Design review of the part shown in the three views and the two pictorial views. Dimensions are in mm from the part's minimum x, y and z. A direction names the side the tool comes from. Coordinates: 2 decimals unless noted, no trailing zeros. Write each loop counter-clockwise with the first axis right and the second up, starting at its lowest first coordinate (ties: lowest second). Pieces come first, ordered by that corner, then holes. Notation, with made-up numbers: (58.5, 37) -> (65.5, 37) arc R9 ccw to (65.5, 50) -> close; hole circle Ø8 at (-6.75, 6). An arc over 180 degrees is marked (long way). Write each question's results on one line, items separated by ' | '.
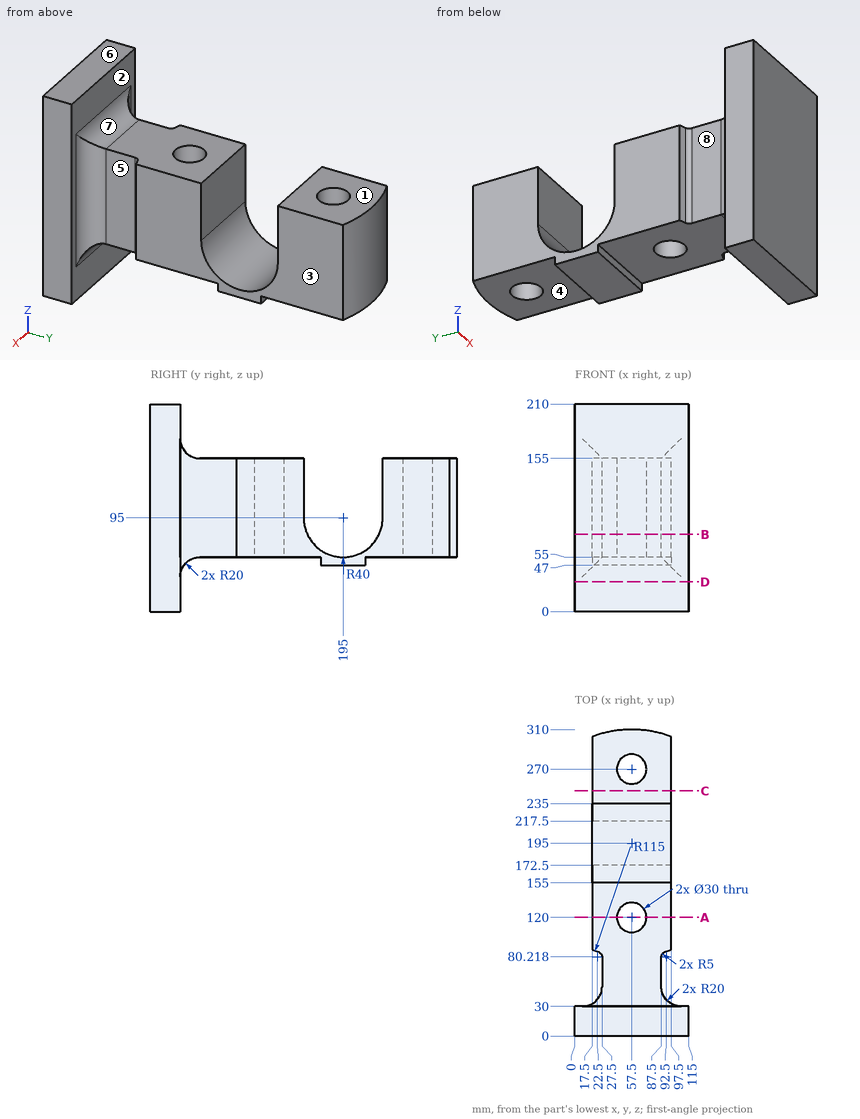
Q1. Add section A-A (y = 120). Write out the cut boundary in (x, z).
Solution:
outline: (17.5, 55) -> (42.5, 55) -> (42.5, 155) -> (17.5, 155) -> close; (72.5, 55) -> (97.5, 55) -> (97.5, 155) -> (72.5, 155) -> close
Q2. Add section D-D (z = 30). Write out the cut boundary in (x, y).
Solution:
outline: (0, 0) -> (115, 0) -> (115, 30) -> (0, 30) -> close
Q3. Machinability: for the marked faces 1, 2, 3, 4 and 5, which of the approach directions +Z, -Z, +X, -X, +Y, -Y give a long, thin tool a straight path to every point of the face, cutting with its end or side? Answer none if there is none.
Solution:
face 1: +Z, +X, -X, +Y | face 2: +Y | face 3: +Z, -Z, +X, +Y | face 4: -Z, +X, -X, +Y | face 5: +Z, -Z, +X
Q4. Draft analysis for pull direction Y (two halves, no side actions). For the marked faces 6, 7 and 8, state which applies: pulls with the +Y half, pulls with the -Y half, needs draft (parallel to the pull), parting line crosses it, or undercut.
Solution:
face 6: needs draft | face 7: pulls with the +Y half | face 8: undercut
Q5. For line 1 (Y direction, x = 57.5, z = 121); line 2 (Y direction, x = 24, z = 100) (1 decimal); line 3 (Y direction, x = 26, z = 65) (1 decimal), list the stretches that pass through material, from the lowest coordinate up. Write a range as from..to.
Solution:
line 1: 0..105, 135..155, 235..255, 285..310 | line 2: 0..38.7, 85..155, 235..305 | line 3: 0..42.4, 83.8..168.5, 221.5..305.6
Q6. Add section B-B (z = 78). Write out the cut boundary in (x, y).
Solution:
outline: (0, 0) -> (115, 0) -> (115, 30) -> (107.5, 30) arc R20 cw to (87.5, 50) -> (87.5, 80.22) arc R5 cw to (91.04, 85) arc R115 ccw to (97.5, 87.18) -> (97.5, 158.79) -> (17.5, 158.79) -> (17.5, 87.18) arc R115 ccw to (23.96, 85) arc R5 cw to (27.5, 80.22) -> (27.5, 50) arc R20 cw to (7.5, 30) -> (0, 30) -> close; (17.5, 231.21) -> (97.5, 231.21) -> (97.5, 302.82) arc R115 ccw to (17.5, 302.82) -> close; hole circle Ø30 at (57.5, 120); hole circle Ø30 at (57.5, 270)
Q7. Add section C-C (y = 248). Write out the cut boundary in (x, z).
Solution:
outline: (17.5, 55) -> (97.5, 55) -> (97.5, 155) -> (17.5, 155) -> close
Q8. Clearance check with flat-ended pins moving along their axes: P1, Ø18, axis at x = 70.5, z = 112.5, coming from the +Y side; P2, Ø4, axis at x = 95.5, y = 242, coming from the -Z side; P3, Ø24, axis at y = 67.5, z = 99.5, coming from the +X side. State where each tip first meets the part, or that it passes through.
Solution:
P1: y = 309.93 | P2: z = 55 | P3: x = 87.5
